Work out the finished part from the listing and answer in its coordinate system (mm). Face numbers are marked on the shaded views. A direction names the side the tool comes from. Coordinates: 2 decimals unless noted, no trailing zeros. Answer as CSV lines item,"result".
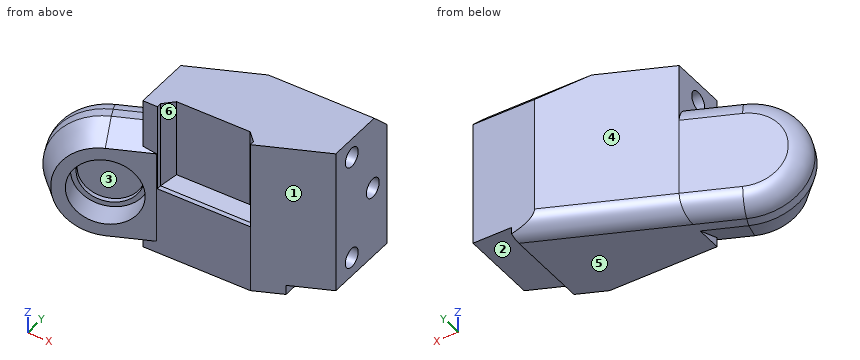
Autodesk Inventor part; units mm, degrees
ref_plane "Work Plane1" through (-20.7027, -4.8012, 0) normal (-0.4001, 0.9165, 0) x (-0.9165, -0.4001, 0)
ref_plane "Work Plane2" through (0, 8, 0) normal (0, 1, 0) x (-1, 0, 0)
ref_plane "YZ Plane" through (0, 0, 0) normal (1, 0, 0) x (0, 1, 0)
sketch "Sketch1" plane through (0, 0, 0) normal (0, 0, 1) x (1, 0, 0)
  line L0 (0, 0) -> (-18, 0) construction
  line L1 (-9.705, 0) -> (-20.7027, -4.8012) construction
  line L2 (-20.7027, -4.8012) -> (-21.1028, -3.8847) construction
  dimension "d0" = 18
  dimension "d1" = 9.705
  dimension "d2" = 23.584
  dimension "d3" = 1
  dimension "d4" = 12
ref_plane "Work Plane1" through (-20.7027, -4.8012, 0) normal (-0.4001, 0.9165, 0) x (-0.9165, -0.4001, 0)
sketch "Sketch3" plane through (-20.7027, -4.8012, 0) normal (-0.4001, 0.9165, 0) x (-0.9165, -0.4001, 0)
  circle A0 centre (0, 0) radius 6
  line L0 (0, -6) -> (-8, -6)
  line L1 (-8, -6) -> (-8, 6)
  line L2 (-8, 6) -> (0, 6)
  line L3 (0, 6) -> (0, -6)
  point P0 (-20.8944, 0)
  point P1 (0, 0)
  dimension "d8" = 12
  dimension "d13" = 8
extrude "Extrusion2" add sketch "Sketch3" along normal blind 6
chamfer "Chamfer2" distance 3 angle 22 3 edges at (-26.2015, -7.2018, 0) (-17.0368, -3.2008, -6) (-17.0368, -3.2008, 6) measured on face at (-26.265, -5.0472, -3) measured on face at (-16.615, -0.8344, 6) measured on face at (-19.0589, -1.9013, -6)
sketch "Sketch2" plane through (0, 0, 0) normal (0, 0, 1) x (1, 0, 0)
  line L0 (-6.8718, -3) -> (-18, -3)
  line L1 (-18, -3) -> (-18, 2.9255)
  line L2 (-18, 2.9255) -> (0, 10.7837)
  line L3 (0, 10.7837) -> (0, 0)
  line L4 (-9.705, 0) -> (-20.7027, -4.8012) construction
  line L5 (-6.8718, -3) -> (0, 0)
  point P0 (0, 0)
  point P1 (-18, 0)
  point P2 (0, 0)
  dimension "d12" = 3
  dimension "d22" = 3
  dimension "d38" = 6
extrude "Extrusion1" add sketch "Sketch2" along normal blind 10 and the other way blind 6
sketch "Sketch5" plane through (-20.7027, -4.8012, 0) normal (0.4001, -0.9165, 0) x (0.9165, 0.4001, 0)
  point P0 (20.8944, 0)
  point P1 (0, 0)
hole "CMC bearing" at (-20.7027, -4.8012, 0) direction (-0.4001, 0.9165, 0) diameter 6 depth 3 counterbore diameter 7 counterbore depth 2.5
sketch "Sketch6" plane through (-18, -3, 10) normal (-1, 0, 0) x (0, 0, 1)
  line L0 (0, 5.9255) -> (0, 0)
  line L1 (0, 5.9255) -> (-4, 5.9255)
  line L2 (0, 0) -> (-4.982, 0)
  line L3 (-2, 5.9255) -> (-2, 0) construction
  point P0 (-10, 3)
  point P1 (-2, 2.9628)
hole "top mount" at (-18, -0.0372, 8) direction (1, 0, 0) diameter 2 depth 8.5
sketch "Sketch8" plane through (-6.8718, -3, -6) normal (0, 0, -1) x (-1, 0, 0)
  line L0 (-6.8718, 3) -> (0, 0)
  line L1 (-6.8718, 13.7837) -> (-6.8718, 3)
  line L2 (16.2314, 3.6976) -> (-6.8718, 13.7837)
  line L3 (-2.8718, 1.2537) -> (-2.8718, 12.0374)
  dimension "d56" = 4
extrude "Extrusion3" cut sketch "Sketch8" against normal blind 1
sketch "Sketch7" plane through (0, 0, 10) normal (1, 0, 0) x (0, 0, -1)
  line L0 (0, 10.7837) -> (15, 10.7837)
  line L1 (0, 0) -> (0, 10.7837)
  line L2 (0, 0) -> (15, 0)
  line L3 (7.5, 0) -> (7.5, 10.7837) construction
  line L4 (15, 0) -> (15, 10.7837)
  point P0 (10, 0)
  point P1 (2, 2.5)
  point P2 (13, 2.5)
  point P3 (7.5, 5.7837)
  dimension "d46" = 5
  dimension "d47" = 11
  dimension "d48" = 2.5
hole "bottom mount" at (0, 2.5, 8) at (0, 5.7837, 2.5) at (0, 2.5, -3) direction (-1, 0, 0) diameter 2 depth 8.5
sketch "Sketch9" plane through (-18, -3, -6) normal (0, -1, 0) x (1, 0, 0)
  line L0 (0, 16) -> (11.1282, 16)
  line L1 (11.1282, 16) -> (1.5, 16)
  line L2 (1.5, 16) -> (1.5, 7)
  line L3 (1.5, 7) -> (11.1282, 7)
  line L4 (11.1282, 7) -> (11.1282, 16)
  point P0 (18, 6)
  dimension "d59" = 9
  dimension "d60" = 1.5
extrude "Extrusion4" cut sketch "Sketch9" against normal blind 1.5
chamfer "Chamfer3" distance 1 angle 45 3 edges at (-16.5, -1.5, 5.5) (-6.8718, -1.5, 5.5) (-11.6859, -1.5, 1)
ref_plane "Work Plane2" through (0, 8, 0) normal (0, 1, 0) x (-1, 0, 0)
split "Split1" plane through (0, 8, 0) removes the side toward (0, 1, 0)
chamfer "Chamfer4" distance 2 angle 45 1 edges at (-3.1882, 8, 10)
fillet "Fillet1" radius 2 3 edges at (-20.5516, 1.8116, 6) (-14.7398, 4.3488, -6) (-28.6021, -1.7029, 0)
equation "\"d2\" = thumb_axis_beta_local"
equation "\"thumb_axis_beta_local\" = thumb_axis_beta"
properties part number "thumb_03 CMC top hinge"
(1) For a pull along X with two mould halves and no side action, classify the marked faces 1, 2, 3 and 4 as pulls with the +X half, pulls with the -X half, needs draft (parallel to the pull), parting line crosses it, or undercut.
Computed values:
face 1,"pulls with the +X half"
face 2,"needs draft"
face 3,"undercut"
face 4,"pulls with the -X half"
(2) Which of the six approach directions +Z, -Z, +X, -X, +Y, -Y give full straight-line access (tool end or side, diameter ignored) to the marked faces 5 and 6?
Computed values:
face 5,"-Z, +X, -X, +Y, -Y"
face 6,"+Z, -Y"
(3) Consider line 1 along Z through (x, y) = (-4.5, 2.5); line 2 along Z through (x, y) = (-2.5, 2.5); line 3 along Z through (x, y) = (-23, -5). Determine where each line is inside the solid, lowest interval first.
Computed values:
line 1,"-6 to -4, -2 to 7, 9 to 10"
line 2,"-5 to -4, -2 to 7, 9 to 10"
line 3,"-4.59 to -2.73, 2.73 to 4.59"
(4) Flat-ended cylindrical pins translate along their axes: pin 1 Ø8 at (x, y) = (-21, 4) entering from -Z; pin 2 Ø0.8 at (y, z) = (-2, -5.5) entering from -X; pin 3 Ø1.6 at (y, z) = (-0.04, 8) entering from -X; pin 4 Ø1.6 at (y, z) = (2, 8.5) entering from +X. Find the tip coordinate at first contact, or state that the pin passes through.
Computed values:
pin 1,"z = -5.99"
pin 2,"x = -25.29"
pin 3,"x = -9.5"
pin 4,"x = 0"
